```python
from build123d import *

# Parameters (mm, degrees)
SKETCH_1_W          = 15
SKETCH_1_H          = 15
SKETCH_1_W_2        = 12
SKETCH_1_H_2        = 12
EXTRUDE_1_DEPTH     = 100
SKETCH_2_R          = 2
CUT_EXTRUDE_1_DEPTH = 102.396498953
SKETCH_3_R          = 3.175
CUT_EXTRUDE_2_DEPTH = 102.396498953


with BuildPart() as part:
    # ｽｹｯﾁ1 → 押し出し-薄板1 (new body)
    with BuildSketch(Plane.XY):
        Rectangle(SKETCH_1_W, SKETCH_1_H)
        Rectangle(SKETCH_1_W_2, SKETCH_1_H_2, mode=Mode.SUBTRACT)
    extrude(amount=EXTRUDE_1_DEPTH)

    # ｽｹｯﾁ2 → ｶｯﾄ - 押し出し1 (cut, through all)
    with BuildSketch(Plane(origin=(7.5, 0, 0), x_dir=(0, 0, -1), z_dir=(1, 0, 0))):
        with Locations(Location((-5, 0, 0), (0, 0, 90))):
            Circle(SKETCH_2_R)
        with Locations(Location((-65, 0, 0), (0, 0, 90))):
            Circle(SKETCH_2_R)
    extrude(amount=-CUT_EXTRUDE_1_DEPTH, mode=Mode.SUBTRACT)

    # ｽｹｯﾁ3 → ｶｯﾄ - 押し出し2 (cut, through all)
    with BuildSketch(Plane(origin=(0, 7.5, 0), x_dir=(1, 0, 0), z_dir=(0, 1, 0))):
        with Locations(Location((0, -85, 0), (0, 0, 180))):
            Circle(SKETCH_3_R)
    extrude(amount=-CUT_EXTRUDE_2_DEPTH, mode=Mode.SUBTRACT)


solid = part.part
```
Geometry check sheet. Reference: the model listing, model coordinates, mm. A direction names the side the tool comes from. Round coordinates to 2 decimals unless told otherwise and drop trailing zeros. Loops run counter-clockwise (first coordinate to the right, second up) from the corner with the lowest first, then second, coordinate; pieces in that order, holes last. Notation, with made-up numbers: M 26,74.5 L 48,74.5 A9 ccw 48,85.5 Z; hole C 75.25,7.25 d6. An arc over 180 degrees is marked long. Return JSON: item names as keys, results as strings. Group by question number.
(1) Set-up check for faces 1 (the face through (-6.74, 1.075, 66.686)), 2 (the face through (0, 6, 49)): record each of +Z, -Z, +X, -X, +Y, -Y from which the full face is reachable in a straight line by a thin tool's end or side.
(2) Section check A-A, the plane z = 39.5. Enter the section's corners in (x, y).
(3) Mould release check, pull along Z, two halves, no side actions. Record for faces 3 (the face through (-7, 0, 100)), 4 (the face through (0.41, -6.74, 88.15)), 5 (the face through (-7, 0, 0)), 6 (the face through (-6, 0, 49)): pulls with the +Z half, pulls with the -Z half, needs draft (parallel to the pull), parting line crosses it, or undercut.
(4) Scan lines: line 1 along Z through (x, y) = (-6.35, 0); line 2 along Y through (x, z) = (4.5, 25). Record each from-to range of solid material in increasing order. Write a range as [from, to].
(5) Go/stop test with a flat-tipped pin: pin 1 (4 mm diameter, centred on x = 0, z = 85, fed in from -Y). Record where the tip stops, or that it passes through.
(6) Section check B-B, the plane y = -5. Enter the section's corners in (x, z).
(7) Section check D-D, the plane y = 0. Enter the section's corners in (x, z), and give its area (3 significant figures).
(8) Section check C-C, the plane x = 0. Enter the section's corners in (y, z) (3 decimals).
Data:
{
 "1": {"face 1": "+X, -X", "face 2": "+Z, -Z"},
 "2": {"outline": "M -7.5,-7.5 L 7.5,-7.5 L 7.5,7.5 L -7.5,7.5 Z; hole M -6,-6 L 6,-6 L 6,6 L -6,6 Z"},
 "3": {"face 3": "pulls with the +Z half", "face 4": "undercut", "face 5": "pulls with the -Z half", "face 6": "needs draft"},
 "4": {"line 1": "[0, 3], [7, 63], [67, 100]", "line 2": "[-7.5, -6], [6, 7.5]"},
 "5": {"pin 1": "through"},
 "6": {"outline": "M -7.5,0 L -6,0 L -6,100 L -7.5,100 Z; M 6,0 L 7.5,0 L 7.5,100 L 6,100 Z"},
 "7": {"outline": "M -7.5,0 L -6,0 L -6,3 L -7.5,3 Z; M -7.5,7 L -6,7 L -6,63 L -7.5,63 Z; M -7.5,67 L -6,67 L -6,100 L -7.5,100 Z; M 6,0 L 7.5,0 L 7.5,3 L 6,3 Z; M 6,7 L 7.5,7 L 7.5,63 L 6,63 Z; M 6,67 L 7.5,67 L 7.5,100 L 6,100 Z", "area": "276 mm²"},
 "8": {"outline": "M -7.5,0 L -6,0 L -6,81.825 L -7.5,81.825 Z; M -7.5,88.175 L -6,88.175 L -6,100 L -7.5,100 Z; M 6,0 L 7.5,0 L 7.5,81.825 L 6,81.825 Z; M 6,88.175 L 7.5,88.175 L 7.5,100 L 6,100 Z"}
}
